For this review, take the finished solid that the model builds, in its own axes (mm). Round coordinates to 2 decimals unless told otherwise and drop trailing zeros. Loops run counter-clockwise (first coordinate to the right, second up) from the corner with the lowest first, then second, coordinate; pieces in that order, holes last.
1) Insertion check: pin 1 (1.5 mm diameter, centred on x = -9, y = -4.5, fed in from -Z); pin 2 (1 mm diameter, centred on x = -12, y = -4, fed in from -Z); pin 3 (10.5 mm diameter, centred on x = -10.01, z = 59.99, fed in from -Y). Each pin has a flat end and moves straight along its axis. Give the tip position at first contact, or say it passes through.
2) Wall thickness on L1, parallel to Z at x = -10.25, y = -1.75; L2, parallel to Z at x = -6.75, y = -7.25; L3, parallel to Z at x = -3.75, y = -6.5: over which ranges is each line inside the solid? List them lowest first.
3) Take a section at C-C (z = -3). State the section outline as (x, y) points, then the cut area to 3 significant figures.
4) Take a section at A-A (x = -9.25). State the section outline as (y, z) points.
5) Take a section at B-B (y = -3.5). State the section outline as (x, z) points.
6) Mouldability with a two-part tool opening along Z and no side actions: class faces 1 (the cylindrical face through (-9.49, -3.94, 63.96)), 2 (the cylindrical face through (-10.228, -3.944, -10.005)), 3 (the flat face through (-20.015, -4, 30)) as pulls with the +Z half, pulls with the -Z half, needs draft (parallel to the pull), parting line crosses it, or undercut.
7) Take a section at D-D (x = -1.5). State the section outline as (y, z) points, then the cut area to 3 significant figures.
```python
from build123d import *

# Parameters (mm, degrees)
F1_DEPTH = 8


with BuildPart() as f1:
    # F0 (on Front) → F1 (new body)
    with BuildSketch(Plane.XZ):
        with BuildLine():
            ThreePointArc((-20.0152, 59.9948), (-10.0076, 49.9872), (0, 59.9948))
            Line((0, 59.9948), (-6.0071, 59.9948))
            ThreePointArc((-6.0071, 59.9948), (-10.0076, 55.9943), (-14.0081, 59.9948))
            Line((-14.0081, 59.9948), (-20.0152, 59.9948))
        make_face()
        with BuildLine():
            Line((-6.0071, 59.9948), (0, 59.9948))
            ThreePointArc((0, 59.9948), (-10.0076, 70.0024), (-20.0152, 59.9948))
            Line((-20.0152, 59.9948), (-14.0081, 59.9948))
            ThreePointArc((-14.0081, 59.9948), (-10.0076, 63.9953), (-6.0071, 59.9948))
        make_face()
        with BuildLine():
            ThreePointArc((-20.0152, 0), (-10.0076, 10.0076), (0, 0))
            Line((0, 0), (0, 59.9948))
            ThreePointArc((0, 59.9948), (-10.0076, 49.9872), (-20.0152, 59.9948))
            Line((-20.0152, 59.9948), (-20.0152, 0))
        make_face()
        with BuildLine():
            ThreePointArc((-20.0152, 0), (-10.0076, -10.0076), (0, 0))
            Line((0, 0), (-6.0071, 0))
            ThreePointArc((-6.0071, 0), (-10.0076, -4.0005), (-14.0081, 0))
            Line((-14.0081, 0), (-20.0152, 0))
        make_face()
        with BuildLine():
            Line((-6.0071, 0), (0, 0))
            ThreePointArc((0, 0), (-10.0076, 10.0076), (-20.0152, 0))
            Line((-20.0152, 0), (-14.0081, 0))
            ThreePointArc((-14.0081, 0), (-10.0076, 4.0005), (-6.0071, 0))
        make_face()
    extrude(amount=F1_DEPTH)


solid = f1.part
```
Response:
1. pin 1: stops at z = -10
1. pin 2: stops at z = -9.9
1. pin 3: stops at y = -8
2. L1: z = -10 to -3.99, 3.99 to 56, 63.99 to 70
2. L2: z = -9.46 to -2.32, 2.32 to 57.67, 62.32 to 69.46
2. L3: z = -7.81 to 67.8
3. outline: (-19.55, -8) - (-12.65, -8) - (-12.65, 0) - (-19.55, 0) - close; (-7.36, -8) - (-0.46, -8) - (-0.46, 0) - (-7.36, 0) - close
3. area: 110 mm2
4. outline: (-8, -9.98) - (0, -9.98) - (0, -3.93) - (-8, -3.93) - close; (-8, 3.93) - (0, 3.93) - (0, 56.07) - (-8, 56.07) - close; (-8, 63.92) - (0, 63.92) - (0, 69.97) - (-8, 69.97) - close
5. outline: (-20.02, 0) arc R10.01 ccw to (0, 0) - (0, 59.99) arc R10.01 ccw to (-20.02, 59.99) - close; hole circle Ø8 at (-10.01, 0); hole circle Ø8 at (-10.01, 59.99)
6. face 1: undercut
6. face 2: pulls with the -Z half
6. face 3: needs draft
7. outline: (-8, -5.27) - (0, -5.27) - (0, 65.26) - (-8, 65.26) - close
7. area: 564 mm2
